```python
from build123d import *

# Parameters (mm, degrees)
SKETCH_1_R                     = 1.5
EXTRUDE_1_DEPTH                = 1.2
SKETCH_2_R                     = 2.25
EXTRUDE_2_DEPTH                = 8
HOLE_WIZARD_M2_5_1_D           = 2.05
HOLE_WIZARD_M2_5_1_CSINK_D     = 2.55
HOLE_WIZARD_M2_5_1_CSINK_ANGLE = 90


with BuildPart() as part:
    # 草图1 → 凸台-拉伸1 (new body)
    with BuildSketch(Plane(origin=(0, 0, 0), x_dir=(1, 0, 0), z_dir=(0, 1, 0))):
        Circle(SKETCH_1_R)
    extrude(amount=EXTRUDE_1_DEPTH)

    # 草图2 → 凸台-拉伸2 (add)
    with BuildSketch(Plane(origin=(0, 1.2, 0), x_dir=(1, 0, 0), z_dir=(0, 1, 0))):
        Circle(SKETCH_2_R)
    extrude(amount=EXTRUDE_2_DEPTH)

    # M2.5 螺纹孔1 (through all)
    with Locations(Plane(origin=(0, 9.2, 0), x_dir=(1, 0, 0), z_dir=(0, 1, 0))):
        with Locations((0, 0)):
            CounterSinkHole(HOLE_WIZARD_M2_5_1_D / 2, HOLE_WIZARD_M2_5_1_CSINK_D / 2, counter_sink_angle=HOLE_WIZARD_M2_5_1_CSINK_ANGLE)


solid = part.part
```
CAD build for the part. Positions are in the model's coordinates, mm. A direction names the side the tool comes from. Round coordinates to 2 decimals unless told otherwise and drop trailing zeros. Order: outer loops, then holes, each group sorted by start corner. A loop starts at its lowest first (then second) coordinate and runs counter-clockwise, first axis right, second up. Notation, with made-up numbers: (68, 56) - (85, 56) arc R24 ccw to (85, 84) - close; hole circle Ø2 at (66.25, 25.5). An arc over 180 degrees is marked (long way). Answer in a Markdown table with one row per item. Add a question column.
(1) Mould opens along Z. For faces 1 (the face through (-0.29, 5.14, -2.23)), 2 (the face through (0.133, 4.412, -1.016)), 3 (the face through (-2, 1.2, 0)) say: +Z half, -Z half, draft (parallel to the pull), parting line (faces both ways), or undercut.
(2) 3-axis set-ups, long thin cutter, end or side, ignore diameter. For faces 4 (the face through (-1.5, 0.59, -0.07)), 5 (the face through (0, 9.2, 1.5)): which of +Z, -Z, +X, -X, +Y, -Y reach the whole face in a straight line?
(3) Drop flat-ended pins along their axis: pin 1 Ø1 at (x, y) = (-1.5, 4) entering from -Z; pin 2 Ø2 at (x, y) = (2, 2.5) entering from +Z. Give the stop position or say it passes through.
(4) Band-saw the part on C-C on y = 1. List the corners of the cut face in (x, z) (3 decimals), and give its area (3 significant figures).
(5) Band-saw the part on D-D on x = -1.7. List the corners of the cut face in (y, z).
(6) Band-saw the part on B-B on z = 0. List the corners of the cut face in (x, y) (3 decimals), and give its area (3 significant figures).
(7) Band-saw the part on A-A on x = 0. List the corners of the cut face in (y, z) (3 decimals).
(8) Probe L1, parallel to Z at x = 0, y = 5.5 (3 decimals); L2, parallel to Y at x = -1.2, z = 1.3; L3, parallel to X at y = 5.25, z = -0.6. List the from-to ranges inside material, lowest first. Write a range as [from, to].
Data:
| question | item | result |
|---|---|---|
| 1 | face 1 | parting line |
| 1 | face 2 | undercut |
| 1 | face 3 | draft |
| 2 | face 4 | -Y |
| 2 | face 5 | +Z, -Z, +X, -X, +Y |
| 3 | pin 1 | stops at z = -2.02 |
| 3 | pin 2 | stops at z = 2.02 |
| 4 | outline | circle Ø3 at (0, 0); hole circle Ø2.05 at (0, 0) |
| 4 | area | 3.77 mm^2 |
| 5 | outline | (1.2, -1.47) - (9.2, -1.47) - (9.2, 1.47) - (1.2, 1.47) - close |
| 6 | outline | (-2.25, 1.2) - (-1.5, 1.2) - (-1.5, 0) - (-1.025, 0) - (-1.025, 8.95) - (-1.275, 9.2) - (-2.25, 9.2) - close; (1.025, 0) - (1.5, 0) - (1.5, 1.2) - (2.25, 1.2) - (2.25, 9.2) - (1.275, 9.2) - (1.025, 8.95) - close |
| 6 | area | 20.7 mm^2 |
| 7 | outline | (0, -1.5) - (1.2, -1.5) - (1.2, -2.25) - (9.2, -2.25) - (9.2, -1.275) - (8.95, -1.025) - (0, -1.025) - close; (0, 1.025) - (8.95, 1.025) - (9.2, 1.275) - (9.2, 2.25) - (1.2, 2.25) - (1.2, 1.5) - (0, 1.5) - close |
| 8 | L1 | z = [-2.25, -1.025], [1.025, 2.25] |
| 8 | L2 | y = [1.2, 9.2] |
| 8 | L3 | x = [-2.17, -0.83], [0.83, 2.17] |
